Part model, mm, in its own coordinate system. A direction names the side the tool comes from. Round coordinates to 2 decimals unless told otherwise and drop trailing zeros. Write each loop counter-clockwise with the first axis right and the second up, starting at its lowest first coordinate (ties: lowest second). Pieces come first, ordered by that corner, then holes. Notation, with made-up numbers: (5.25, -6) -> (40.25, -6) arc R8 ccw to (40.25, 4) -> close; hole circle Ø3 at (62, 43.25). An arc over 180 degrees is marked (long way). Use CSV: the item, a comma, the result in double quotes. Start each with the question number.
```python
from build123d import *

# Parameters (mm, degrees)
BOSS_EXTRUDE1_DEPTH = 5
SKETCH2_R           = 3
CUT_EXTRUDE1_DEPTH  = 10


with BuildPart() as part:
    # Sketch1 → Boss-Extrude1 (new body)
    with BuildSketch(Plane(origin=(0, 0, 0), x_dir=(1, 0, 0), z_dir=(0, 1, 0))):
        Polygon((-10, 20), (-10, -20), (-3.5, -20), (-3.5, -15), (3.5, -15), (3.5, -20), (10, -20), (10, 20), (3.5, 20), (3.5, 25), (-3.5, 25), (-3.5, 20), align=None)
    extrude(amount=BOSS_EXTRUDE1_DEPTH)

    # Sketch2 → Cut-Extrude1 (cut)
    with BuildSketch(Plane(origin=(0, 5, 0), x_dir=(1, 0, 0), z_dir=(0, 1, 0))):
        with Locations(Location((0, -2.5, 0), (0, 0, 270))):
            Circle(SKETCH2_R)
    extrude(amount=-CUT_EXTRUDE1_DEPTH, mode=Mode.SUBTRACT)


solid = part.part
```
1. Band-saw the part on B-B (x = 0). List the corners of the cut face in (y, z), then the cut area to 3 significant figures.
2. Which spindle directions (+Z, -Z, +X, -X, +Y, -Y) get a long thin tool onto all of the face, cutting with end or side? Do faces 4 (the flat face through (0, 2, 15)), 5 (the flat face through (7, 2, -20)), 6 (the flat face through (-3.5, 2, -23)), 7 (the flat face through (-7, 2, 20)). Say none if no direction does.
3. Band-saw the part on D-D (x = 5.5). List the corners of the cut face in (y, z), then the cut area to 3 significant figures.
4. Drill centre lines: line 1 along X through (y, z) = (3.6, 17.5); line 2 along Z through (x, y) = (-4.5, 3.95); line 3 along Z through (x, y) = (-2.75, 2.8). Where is each one in solid material? Low to high. Write a range as [from, to].
5. Band-saw the part on A-A (z = 2.5). List the corners of the cut face in (x, y), then the cut area to 3 significant figures.
6. Pull direction X, two halves, no side cores. Call faces 1 (the flat face through (0, 2, -25)), 2 (the flat face through (3.5, 2, -22)), 3 (the flat face through (3.5, 2, 17)): released by +X, released by -X, zero draft, split by the parting line, or undercut.
7. Flat gauge pins, fed straight in: pin 1 (2.5 mm diameter, centred on y = 2.5, z = -23.5, fed in from +X); pin 2 (2.5 mm diameter, centred on x = 6, y = 3, fed in from -Z); pin 3 (3 mm diameter, centred on x = 0, y = 3.5, fed in from +Z). Where does each tip first touch, or does it go through?
8. Band-saw the part on C-C (y = 1.5). List the corners of the cut face in (x, z), then the cut area to 3 significant figures.
Answers below:
1,outline,"(0, -25) -> (5, -25) -> (5, -0.5) -> (0, -0.5) -> close; (0, 5.5) -> (5, 5.5) -> (5, 15) -> (0, 15) -> close"
1,area,"170 mm^2"
2,face 4,"+Z, +Y, -Y"
2,face 5,"-Z, +X, +Y, -Y"
2,face 6,"-Z, -X, +Y, -Y"
2,face 7,"+Z, +X, -X, +Y, -Y"
3,outline,"(0, -20) -> (5, -20) -> (5, 20) -> (0, 20) -> close"
3,area,"200 mm^2"
4,line 1,"x = [-10, -3.5], [3.5, 10]"
4,line 2,"z = [-20, 20]"
4,line 3,"z = [-25, 1.3], [3.7, 15]"
5,outline,"(-10, 0) -> (-3, 0) -> (-3, 5) -> (-10, 5) -> close; (3, 0) -> (10, 0) -> (10, 5) -> (3, 5) -> close"
5,area,"70.0 mm^2"
6,face 1,"zero draft"
6,face 2,"released by +X"
6,face 3,"undercut"
7,pin 1,"stops at x = 3.5"
7,pin 2,"stops at z = -20"
7,pin 3,"stops at z = 15"
8,outline,"(-10, -20) -> (-3.5, -20) -> (-3.5, -25) -> (3.5, -25) -> (3.5, -20) -> (10, -20) -> (10, 20) -> (3.5, 20) -> (3.5, 15) -> (-3.5, 15) -> (-3.5, 20) -> (-10, 20) -> close; hole circle Ø6 at (0, 2.5)"
8,area,"772 mm^2"
